Verification items for the finished model (mm, model axes). Face numbers are marked on the shaded views. Give positions to 0.01 mm unless a question says otherwise; leave off trailing zeros. Loops run counter-clockwise (first coordinate to the right, second up) from the corner with the lowest first, then second, coordinate; pieces in that order, holes last. Notation, with made-up numbers: (-29, 89) - (17, 89) arc R20 cw to (17, 122) - close; hole circle Ø8 at (15.25, 31.25). An arc over 180 degrees is marked (long way). Answer in a Markdown table with one row per item.
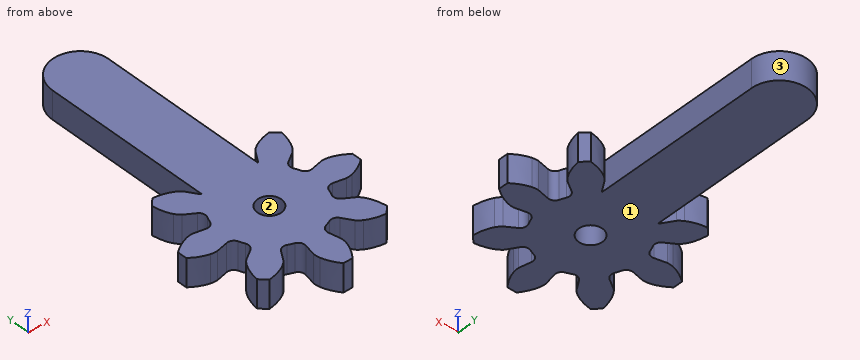
```python
from build123d import *

# Parameters (mm, degrees)
CYLINDER008_R     = 1.7
CYLINDER008_DEPTH = 10
EXTRUDE019_DEPTH  = 4
EXTRUDE021_DEPTH  = 4


with BuildPart() as cylinder008:
    # Cylinder008 → Cylinder008 (new body)
    with BuildSketch(Plane(origin=(21, 0, -4), x_dir=(1, 0, 0), z_dir=(0, 0, 1))):
        Circle(CYLINDER008_R)
    extrude(amount=CYLINDER008_DEPTH)


with BuildPart() as extrude019:
    # InvoluteGear006 → Extrude019 (new body)
    with BuildSketch(Plane.XY):
        with BuildLine():
            Line((7.583619, -1.626335), (9.226112, -1.976129))
            add(Edge.make_bspline(
                [(9.226112, -1.976129), (9.323588, -1.988042), (9.615448, -2.006593), (10.112858, -1.891348)],
                knots=[0, 0, 0, 0, 1, 1, 1, 1], degree=3))
            add(Edge.make_bspline(
                [(10.112858, -1.891348), (10.701098, -1.749257), (11.528547, -1.419904), (12.486309, -0.674071)],
                knots=[0, 0, 0, 0, 1, 1, 1, 1], degree=3))
            ThreePointArc((12.486309, -0.674071), (12.504498, 0), (12.486309, 0.674071))
            add(Edge.make_bspline(
                [(12.486309, 0.674071), (11.528547, 1.419904), (10.701098, 1.749257), (10.112858, 1.891348)],
                knots=[0, 0, 0, 0, 1, 1, 1, 1], degree=3))
            add(Edge.make_bspline(
                [(10.112858, 1.891348), (9.615448, 2.006593), (9.323588, 1.988042), (9.226112, 1.976129)],
                knots=[0, 0, 0, 0, 1, 1, 1, 1], degree=3))
            Line((9.226112, 1.976129), (7.583619, 1.626335))
            ThreePointArc((7.583619, 1.626335), (6.928673, 1.725171), (6.502518, 2.232237))
            ThreePointArc((6.502518, 2.232237), (6.351672, 2.630949), (6.176404, 3.019545))
            ThreePointArc((6.176404, 3.019545), (6.119192, 3.679432), (6.512421, 4.212436))
            Line((6.512421, 4.212436), (7.92118, 5.126512))
            add(Edge.make_bspline(
                [(7.92118, 5.126512), (7.99853, 5.187015), (8.218024, 5.380273), (8.488255, 5.813485)],
                knots=[0, 0, 0, 0, 1, 1, 1, 1], degree=3))
            add(Edge.make_bspline(
                [(8.488255, 5.813485), (8.803731, 6.329908), (9.155937, 7.14789), (9.305795, 8.352514)],
                knots=[0, 0, 0, 0, 1, 1, 1, 1], degree=3))
            ThreePointArc((9.305795, 8.352514), (8.842015, 8.842015), (8.352514, 9.305795))
            add(Edge.make_bspline(
                [(8.352514, 9.305795), (7.14789, 9.155937), (6.329908, 8.803731), (5.813485, 8.488255)],
                knots=[0, 0, 0, 0, 1, 1, 1, 1], degree=3))
            add(Edge.make_bspline(
                [(5.813485, 8.488255), (5.380273, 8.218024), (5.187015, 7.99853), (5.126512, 7.92118)],
                knots=[0, 0, 0, 0, 1, 1, 1, 1], degree=3))
            Line((5.126512, 7.92118), (4.212436, 6.512421))
            ThreePointArc((4.212436, 6.512421), (3.679432, 6.119192), (3.019545, 6.176404))
            ThreePointArc((3.019545, 6.176404), (2.630949, 6.351672), (2.232237, 6.502518))
            ThreePointArc((2.232237, 6.502518), (1.725171, 6.928673), (1.626335, 7.583619))
            Line((1.626335, 7.583619), (1.976129, 9.226112))
            add(Edge.make_bspline(
                [(1.976129, 9.226112), (1.988042, 9.323588), (2.006593, 9.615448), (1.891348, 10.112858)],
                knots=[0, 0, 0, 0, 1, 1, 1, 1], degree=3))
            add(Edge.make_bspline(
                [(1.891348, 10.112858), (1.749257, 10.701098), (1.419904, 11.528547), (0.674071, 12.486309)],
                knots=[0, 0, 0, 0, 1, 1, 1, 1], degree=3))
            ThreePointArc((0.674071, 12.486309), (0, 12.504498), (-0.674071, 12.486309))
            add(Edge.make_bspline(
                [(-0.674071, 12.486309), (-1.419904, 11.528547), (-1.749257, 10.701098), (-1.891348, 10.112858)],
                knots=[0, 0, 0, 0, 1, 1, 1, 1], degree=3))
            add(Edge.make_bspline(
                [(-1.891348, 10.112858), (-2.006593, 9.615448), (-1.988042, 9.323588), (-1.976129, 9.226112)],
                knots=[0, 0, 0, 0, 1, 1, 1, 1], degree=3))
            Line((-1.976129, 9.226112), (-1.626335, 7.583619))
            ThreePointArc((-1.626335, 7.583619), (-1.725171, 6.928673), (-2.232237, 6.502518))
            ThreePointArc((-2.232237, 6.502518), (-2.630949, 6.351672), (-3.019545, 6.176404))
            ThreePointArc((-3.019545, 6.176404), (-3.679432, 6.119192), (-4.212436, 6.512421))
            Line((-4.212436, 6.512421), (-5.126512, 7.92118))
            add(Edge.make_bspline(
                [(-5.126512, 7.92118), (-5.187015, 7.99853), (-5.380273, 8.218024), (-5.813485, 8.488255)],
                knots=[0, 0, 0, 0, 1, 1, 1, 1], degree=3))
            add(Edge.make_bspline(
                [(-5.813485, 8.488255), (-6.329908, 8.803731), (-7.14789, 9.155937), (-8.352514, 9.305795)],
                knots=[0, 0, 0, 0, 1, 1, 1, 1], degree=3))
            ThreePointArc((-8.352514, 9.305795), (-8.842015, 8.842015), (-9.305795, 8.352514))
            add(Edge.make_bspline(
                [(-9.305795, 8.352514), (-9.155937, 7.14789), (-8.803731, 6.329908), (-8.488255, 5.813485)],
                knots=[0, 0, 0, 0, 1, 1, 1, 1], degree=3))
            add(Edge.make_bspline(
                [(-8.488255, 5.813485), (-8.218024, 5.380273), (-7.99853, 5.187015), (-7.92118, 5.126512)],
                knots=[0, 0, 0, 0, 1, 1, 1, 1], degree=3))
            Line((-7.92118, 5.126512), (-6.512421, 4.212436))
            ThreePointArc((-6.512421, 4.212436), (-6.119192, 3.679432), (-6.176404, 3.019545))
            ThreePointArc((-6.176404, 3.019545), (-6.351672, 2.630949), (-6.502518, 2.232237))
            ThreePointArc((-6.502518, 2.232237), (-6.928673, 1.725171), (-7.583619, 1.626335))
            Line((-7.583619, 1.626335), (-9.226112, 1.976129))
            add(Edge.make_bspline(
                [(-9.226112, 1.976129), (-9.323588, 1.988042), (-9.615448, 2.006593), (-10.112858, 1.891348)],
                knots=[0, 0, 0, 0, 1, 1, 1, 1], degree=3))
            add(Edge.make_bspline(
                [(-10.112858, 1.891348), (-10.701098, 1.749257), (-11.528547, 1.419904), (-12.486309, 0.674071)],
                knots=[0, 0, 0, 0, 1, 1, 1, 1], degree=3))
            ThreePointArc((-12.486309, 0.674071), (-12.504498, 0), (-12.486309, -0.674071))
            add(Edge.make_bspline(
                [(-12.486309, -0.674071), (-11.528547, -1.419904), (-10.701098, -1.749257), (-10.112858, -1.891348)],
                knots=[0, 0, 0, 0, 1, 1, 1, 1], degree=3))
            add(Edge.make_bspline(
                [(-10.112858, -1.891348), (-9.615448, -2.006593), (-9.323588, -1.988042), (-9.226112, -1.976129)],
                knots=[0, 0, 0, 0, 1, 1, 1, 1], degree=3))
            Line((-9.226112, -1.976129), (-7.583619, -1.626335))
            ThreePointArc((-7.583619, -1.626335), (-6.928673, -1.725171), (-6.502518, -2.232237))
            ThreePointArc((-6.502518, -2.232237), (-6.351672, -2.630949), (-6.176404, -3.019545))
            ThreePointArc((-6.176404, -3.019545), (-6.119192, -3.679432), (-6.512421, -4.212436))
            Line((-6.512421, -4.212436), (-7.92118, -5.126512))
            add(Edge.make_bspline(
                [(-7.92118, -5.126512), (-7.99853, -5.187015), (-8.218024, -5.380273), (-8.488255, -5.813485)],
                knots=[0, 0, 0, 0, 1, 1, 1, 1], degree=3))
            add(Edge.make_bspline(
                [(-8.488255, -5.813485), (-8.803731, -6.329908), (-9.155937, -7.14789), (-9.305795, -8.352514)],
                knots=[0, 0, 0, 0, 1, 1, 1, 1], degree=3))
            ThreePointArc((-9.305795, -8.352514), (-8.842015, -8.842015), (-8.352514, -9.305795))
            add(Edge.make_bspline(
                [(-8.352514, -9.305795), (-7.14789, -9.155937), (-6.329908, -8.803731), (-5.813485, -8.488255)],
                knots=[0, 0, 0, 0, 1, 1, 1, 1], degree=3))
            add(Edge.make_bspline(
                [(-5.813485, -8.488255), (-5.380273, -8.218024), (-5.187015, -7.99853), (-5.126512, -7.92118)],
                knots=[0, 0, 0, 0, 1, 1, 1, 1], degree=3))
            Line((-5.126512, -7.92118), (-4.212436, -6.512421))
            ThreePointArc((-4.212436, -6.512421), (-3.679432, -6.119192), (-3.019545, -6.176404))
            ThreePointArc((-3.019545, -6.176404), (-2.630949, -6.351672), (-2.232237, -6.502518))
            ThreePointArc((-2.232237, -6.502518), (-1.725171, -6.928673), (-1.626335, -7.583619))
            Line((-1.626335, -7.583619), (-1.976129, -9.226112))
            add(Edge.make_bspline(
                [(-1.976129, -9.226112), (-1.988042, -9.323588), (-2.006593, -9.615448), (-1.891348, -10.112858)],
                knots=[0, 0, 0, 0, 1, 1, 1, 1], degree=3))
            add(Edge.make_bspline(
                [(-1.891348, -10.112858), (-1.749257, -10.701098), (-1.419904, -11.528547), (-0.674071, -12.486309)],
                knots=[0, 0, 0, 0, 1, 1, 1, 1], degree=3))
            ThreePointArc((-0.674071, -12.486309), (0, -12.504498), (0.674071, -12.486309))
            add(Edge.make_bspline(
                [(0.674071, -12.486309), (1.419904, -11.528547), (1.749257, -10.701098), (1.891348, -10.112858)],
                knots=[0, 0, 0, 0, 1, 1, 1, 1], degree=3))
            add(Edge.make_bspline(
                [(1.891348, -10.112858), (2.006593, -9.615448), (1.988042, -9.323588), (1.976129, -9.226112)],
                knots=[0, 0, 0, 0, 1, 1, 1, 1], degree=3))
            Line((1.976129, -9.226112), (1.626335, -7.583619))
            ThreePointArc((1.626335, -7.583619), (1.725171, -6.928673), (2.232237, -6.502518))
            ThreePointArc((2.232237, -6.502518), (2.630949, -6.351672), (3.019545, -6.176404))
            ThreePointArc((3.019545, -6.176404), (3.679432, -6.119192), (4.212436, -6.512421))
            Line((4.212436, -6.512421), (5.126512, -7.92118))
            add(Edge.make_bspline(
                [(5.126512, -7.92118), (5.187015, -7.99853), (5.380273, -8.218024), (5.813485, -8.488255)],
                knots=[0, 0, 0, 0, 1, 1, 1, 1], degree=3))
            add(Edge.make_bspline(
                [(5.813485, -8.488255), (6.329908, -8.803731), (7.14789, -9.155937), (8.352514, -9.305795)],
                knots=[0, 0, 0, 0, 1, 1, 1, 1], degree=3))
            ThreePointArc((8.352514, -9.305795), (8.842015, -8.842015), (9.305795, -8.352514))
            add(Edge.make_bspline(
                [(9.305795, -8.352514), (9.155937, -7.14789), (8.803731, -6.329908), (8.488255, -5.813485)],
                knots=[0, 0, 0, 0, 1, 1, 1, 1], degree=3))
            add(Edge.make_bspline(
                [(8.488255, -5.813485), (8.218024, -5.380273), (7.99853, -5.187015), (7.92118, -5.126512)],
                knots=[0, 0, 0, 0, 1, 1, 1, 1], degree=3))
            Line((7.92118, -5.126512), (6.512421, -4.212436))
            ThreePointArc((6.512421, -4.212436), (6.119192, -3.679432), (6.176404, -3.019545))
            ThreePointArc((6.176404, -3.019545), (6.351672, -2.630949), (6.502518, -2.232237))
            ThreePointArc((6.502518, -2.232237), (6.928673, -1.725171), (7.583619, -1.626335))
        make_face()
    extrude(amount=EXTRUDE019_DEPTH)


with BuildPart() as extrude019_1:
    # Extrude019 placement: moved
    add(extrude019.part.moved(Location((21, 0, 0))))


with BuildPart() as cut007:
    # Sketch012 → Extrude021 (new body)
    with BuildSketch(Plane.XY):
        with BuildLine():
            ThreePointArc((-4, 0), (0, -4), (4, 0))
            Line((4, 0), (4, 30))
            ThreePointArc((4, 30), (0, 34), (-4, 30))
            Line((-4, 0), (-4, 30))
        make_face()
    extrude(amount=EXTRUDE021_DEPTH)


with BuildPart() as cut007_1:
    # Extrude021 placement: moved
    add(cut007.part.moved(Location((21, 0, 0))))

    # Fusion005: union Extrude019
    add(extrude019_1.part)

    # Cut007: cut Cylinder008
    add(cylinder008.part, mode=Mode.SUBTRACT)


with BuildPart() as cut007_2:
    # Cut007 placement: moved
    add(cut007_1.part.moved(Location((0, 0, 31))))


solid = cut007_2.part
```
Q1. Draft check along Y on the marked faces 1, 2 and 3. Enter one of: +Y half, -Y half, draft (parallel to the pull), parting line (faces both ways), or undercut.
Completed:
| item | result |
|---|---|
| face 1 | draft |
| face 2 | undercut |
| face 3 | +Y half |
Q2. Sectioned sample at A-A (x = 21). Record the cut outline in (y, z).
Completed:
| item | result |
|---|---|
| outline | (-12.5, 31) - (-1.7, 31) - (-1.7, 35) - (-12.5, 35) - close; (1.7, 31) - (34, 31) - (34, 35) - (1.7, 35) - close |
Q3. Sectioned sample at C-C (y = 23.5). Record the cut outline in (x, z).
Completed:
| item | result |
|---|---|
| outline | (17, 31) - (25, 31) - (25, 35) - (17, 35) - close |
Q4. Thickness scan on line 1 (Y direction, x = 21, z = 32.6); line 2 (Y direction, x = 29.75, z = 34.35); line 3 (Y direction, x = 28.5, z = 34.4). Record the ranges inside material, lowest first.
Completed:
| item | result |
|---|---|
| line 1 | -12.5 to -1.7, 1.7 to 34 |
| line 2 | -8.93 to -6.31, -1.87 to 1.87, 6.31 to 8.93 |
| line 3 | -9.15 to -4.85, -1.61 to 1.61, 4.85 to 9.15 |
Q5. Sectioned sample at B-B (y = 0). Record the cut outline in (x, z).
Completed:
| item | result |
|---|---|
| outline | (8.5, 31) - (19.3, 31) - (19.3, 35) - (8.5, 35) - close; (22.7, 31) - (33.5, 31) - (33.5, 35) - (22.7, 35) - close |
